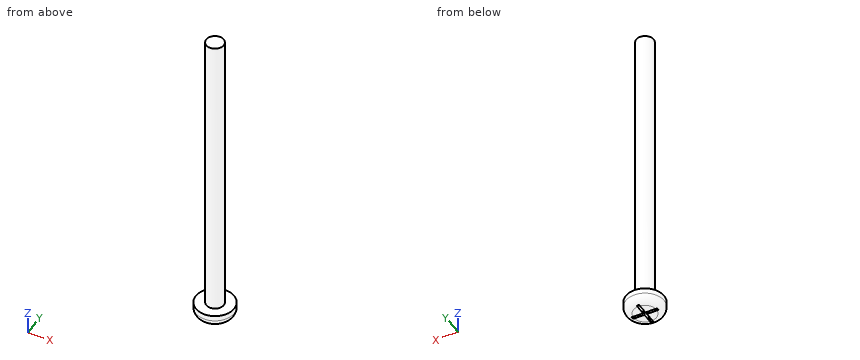
```python
from build123d import *

# Parameters (mm, degrees)
SKETCH_1_R               = 1.75
EXTRUDE_1_DEPTH          = 1.2
SKETCH_2_R               = 0.8
EXTRUDE_2_DEPTH          = 27.4
PATTERN_CIRCULAR_1_COUNT = 4
FILLET_2_R               = 0.7


with BuildPart() as part:
    # 草圖1 → 伸長1 (new body)
    with BuildSketch(Plane.XY):
        Circle(SKETCH_1_R)
    extrude(amount=EXTRUDE_1_DEPTH)

    # 草圖2 → 伸長2 (add)
    with BuildSketch(Plane.XY.offset(1.2)):
        with Locations(Location((0, 0, 0), (0, 0, 180))):
            Circle(SKETCH_2_R)
    extrude(amount=EXTRUDE_2_DEPTH)

    # 草圖3 → 除料-疊層拉伸1 section 0
    with BuildSketch(Plane(origin=(0, 0, 0), x_dir=(-1, 0, 0), z_dir=(0, 0, -1)), mode=Mode.PRIVATE) as loft_1_s0:
        with BuildLine():
            Line((-0.115, 1.2), (0.115, 1.2))
            Line((0.115, 1.2), (0.115, -1.2))
            Line((0.115, -1.2), (-0.115, -1.2))
            Line((-0.115, -1.2), (-0.115, 1.2))
        make_face()
    loft_1 = loft([loft_1_s0.sketch, Vertex(0, 0, 0.85)], mode=Mode.SUBTRACT)

    # 環狀複製排列1: 除料-疊層拉伸1 ×4 about axis
    pattern_circular_1_axis = Axis((0, 0, 0), (0, 0, 1))
    for i in range(1, PATTERN_CIRCULAR_1_COUNT):
        add(loft_1.rotate(pattern_circular_1_axis, i * 360 / PATTERN_CIRCULAR_1_COUNT), mode=Mode.SUBTRACT)

    # 圓角2
    # the kernel refuses this fillet: 0.7 mm, written as the material it takes off along each edge
    with BuildSketch(Plane(origin=(0, 0, 0), x_dir=(1, 0, 0), z_dir=(0, -1, 0))) as fillet_2_piece_1:
        with BuildLine():
            CenterArc((1.75 - FILLET_2_R, FILLET_2_R), FILLET_2_R, 270, 90)
            Line((1.75 - FILLET_2_R, 0), (1.75, 0))
            Line((1.75, 0), (1.75, FILLET_2_R))
        make_face()
    revolve(axis=Axis((0, 0, 0), (0, 0, 1)), mode=Mode.SUBTRACT)


solid = part.part
```
The model under review builds one solid part; all positions refer to its coordinate system, in mm. Coordinates: 2 decimals unless noted, no trailing zeros. Write each loop counter-clockwise with the first axis right and the second up, starting at its lowest first coordinate (ties: lowest second). Pieces come first, ordered by that corner, then holes. Notation, with made-up numbers: (-34.75, 74) - (9.25, 74) arc R17 ccw to (9.25, 106) - close; hole circle Ø9 at (17.25, 26.25). An arc over 180 degrees is marked (long way). Answer in a Markdown table with one row per item. Add a question column.
Q1. To check wall thickness, follow line 1 along Z through (x, y) = (-0.7, -0.65); line 2 along Y through (x, z) = (-0.1, 13.5); line 3 along Y through (x, z) = (-0.55, 21). State the ranges of each line that lie inside material, in increasing order. Write a range as from..to.
Q2. Consider section A-A on z = 23.25. Give the boundary of the cut face in (x, y).
Q3. Clearance check with a flat-ended pin moving along its axis: pin 1 (2 mm diameter, centred on y = 1, z = 3, fed in from -X). State where the tip first meets the part, or that it passes through.
Answers below:
| question | item | result |
|---|---|---|
| 1 | line 1 | 0..1.2 |
| 1 | line 2 | -0.79..0.79 |
| 1 | line 3 | -0.58..0.58 |
| 2 | outline | circle Ø1.6 at (0, 0) |
| 3 | pin 1 | x = -0.8 |
